Can you work these out from the model? Positions are in its coordinate system, mm. Face numbers are marked on the shaded views. A direction names the side the tool comes from. Give positions to 0.01 mm unless a question says otherwise; leave off trailing zeros. Loops run counter-clockwise (first coordinate to the right, second up) from the corner with the lowest first, then second, coordinate; pieces in that order, holes last. Notation, with made-up numbers: (67, 82) - (119, 82) arc R20 cw to (119, 91) - close; hole circle Ø1 at (65, 10.25). An arc over 180 degrees is marked (long way). Answer as a JSON object with one key per item and string values.
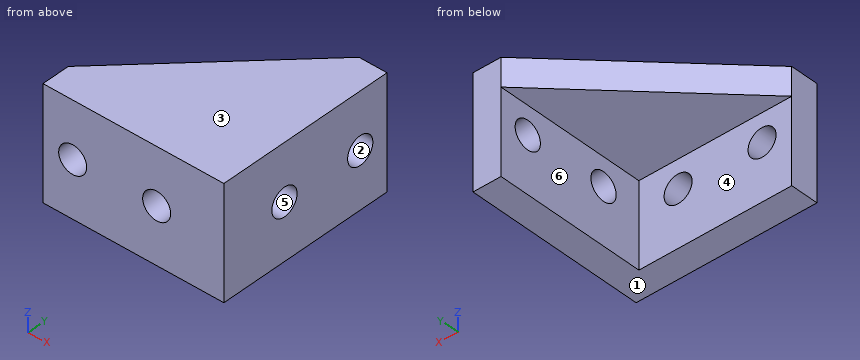
Autodesk Inventor part; units mm, degrees
ref_plane "YZ Plane" through (0, 0, 0) normal (1, 0, 0) x (0, 1, 0)
ref_plane "XZ Plane" through (0, 0, 0) normal (0, 1, 0) x (-1, 0, 0)
ref_plane "XY Plane" through (0, 0, 0) normal (0, 0, 1) x (1, 0, 0)
sketch "Sketch1" plane through (0, 0, 0) normal (0, 0, 1) x (1, 0, 0)
  line L0 (0, 0) -> (50, 0)
  line L1 (50, 0) -> (50, 50)
  line L2 (50, 50) -> (0, 0)
  dimension "d0" = 50
  dimension "d1" = 50
extrude "Extrusion1" add sketch "Sketch1" along normal blind 20
sketch "Sketch2" plane through (0, 0, 20) normal (0, 0, 1) x (1, 0, 0)
  line L0 (50, 50) -> (0, 0)
  line L1 (5, 5) -> (45, 5)
  line L2 (45, 5) -> (45, 45)
  line L3 (50, 0) -> (50, 50)
  line L4 (0, 0) -> (50, 0)
  dimension "d4" = 5
  dimension "d5" = 5
extrude "Extrusion2" cut sketch "Sketch2" against normal through all contours L2 L1 L0
extrude "Extrusion3" add sketch "Sketch2" against normal blind 5 contours L2 L1 L0
sketch "Sketch3" plane through (0, 0, 0) normal (0, 0, -1) x (-1, 0, 0)
  line L0 (-12.7, 0) -> (-50, 37.3)
  line L1 (-50, 0) -> (-50, 50)
  line L2 (-60.6675, 53.6604) -> (-50, 37.3)
  line L3 (-60.6675, 53.6604) -> (-37.4752, 61.571)
  line L4 (-37.4752, 61.571) -> (23.8314, -5.4888)
  line L5 (23.8314, -5.4888) -> (-5.9204, -12.6802)
  line L6 (-5.9204, -12.6802) -> (-12.7, 0)
  point P0 (0, 0)
  dimension "d12" = 12.7
  dimension "d13" = 12.7
extrude "Extrusion5" cut sketch "Sketch3" against normal through all
sketch "Sketch5" plane through (45, 5, 0) normal (-1, 0, 0) x (0, 0, 1)
  line L0 (0, 0) -> (0, 27.3)
  line L1 (20, -5) -> (0, -5)
  point P0 (10, 22)
  point P1 (10, 7)
  dimension "d28" = 10
  dimension "d29" = 10
  dimension "d30" = 15
  dimension "d31" = 12
hole "Hole2" at (45, 27, 10) at (45, 12, 10) direction (1, 0, 0) diameter 5 depth 25.4 tip angle 118
sketch "Sketch6" plane through (45, 5, 15) normal (0, 1, 0) x (1, 0, 0)
  line L0 (-27.3, 15) -> (0, 15)
  line L1 (5, 15) -> (5, -5)
  point P0 (-45, 15)
  point P1 (-7, 5)
  point P2 (-22, 5)
  dimension "d39" = 15
  dimension "d40" = 10
  dimension "d41" = 10
  dimension "d42" = 12
hole "Hole3" at (38, 5, 10) at (23, 5, 10) direction (0, -1, 0) diameter 5 depth 25.4 tip angle 118
sketch "Sketch7" plane through (0, 0, 0) normal (0, 0, -1) x (-1, 0, 0)
  line L0 (-17.7, 5) -> (-17.7, 0)
  line L1 (-12.7, 0) -> (-50, 0)
  line L2 (-17.7, 0) -> (-12.7, 0)
  line L3 (-12.7, 0) -> (-17.7, 5)
  line L4 (-12.7, 0) -> (-17.7, 5)
  line L5 (-45, 32.3) -> (-50, 32.3)
  line L6 (-50, 0) -> (-50, 37.3)
  line L7 (-50, 32.3) -> (-50, 37.3)
  line L8 (-50, 37.3) -> (-45, 32.3)
  line L9 (-45, 32.3) -> (-50, 37.3)
  point P0 (0, 0)
extrude "Extrusion6" cut sketch "Sketch7" against normal blind 25.4
properties part number "corners"
1) Imagine slicing it at C-C on z = 9.5. Write out the boundary of the cut face in (x, y).
Check sheet entries:
{"outline": "(17.7, 0) - (20.55, 0) - (20.55, 5) - (17.7, 5) - close; (25.45, 0) - (35.55, 0) - (35.55, 5) - (25.45, 5) - close; (40.45, 0) - (50, 0) - (50, 9.55) - (45, 9.55) - (45, 5) - (40.45, 5) - close; (45, 14.45) - (50, 14.45) - (50, 24.55) - (45, 24.55) - close; (45, 29.45) - (50, 29.45) - (50, 32.3) - (45, 32.3) - close"}
2) Imagine slicing it at B-B on x = 38. Write out the boundary of the cut face in (y, z).
Check sheet entries:
{"outline": "(0, 0) - (5, 0) - (5, 7.5) - (0, 7.5) - close; (0, 12.5) - (5, 12.5) - (5, 15) - (25.3, 15) - (25.3, 20) - (0, 20) - close"}
3) I'm going to push flat-ended pins straight in: P1, Ø6, axis at y = 16.5, z = 6.5, coming from the -X side; P2, Ø1.5, axis at x = 24.5, y = 12.5, coming from the -Z side; P3, Ø12, axis at y = 18.5, z = 17.5, coming from the -X side. Where does each tip first touch, or does it pass through?
Check sheet entries:
{"P1": "x = 45", "P2": "z = 15", "P3": "x = 25.2"}
4) I need wall thicknesses on L1, parallel to X at y = 3.6, z = 10; L2, parallel to Y at x = 46.95, z = 10; L3, parallel to Z at x = 47.75, y = 12. Which ranges of each line are inside material? Lowest first, please.
Check sheet entries:
{"L1": "17.7 to 20.5, 25.5 to 35.5, 40.5 to 50", "L2": "0 to 9.5, 14.5 to 24.5, 29.5 to 32.3", "L3": "0 to 7.5, 12.5 to 20"}
5) Which directions (+Z, -Z, +X, -X, +Y, -Y) give clear straight access to the entire face, cutting with the end or side of a thin tool? Please do the marked faces 5 and 6.
Check sheet entries:
{"face 5": "+X, -X", "face 6": "-Z, -X, +Y"}
6) If we mould it in two halves opening along Z, with no side actions, what happens to the marked faces 1, 2, 3 and 4? For each: released by +Z, released by -Z, zero draft, split by the parting line, or undercut.
Check sheet entries:
{"face 1": "released by -Z", "face 2": "undercut", "face 3": "released by +Z", "face 4": "zero draft"}
7) Imagine slicing it at A-A on y = 29. Write out the boundary of the cut face in (x, z).
Check sheet entries:
{"outline": "(41.7, 15) - (45, 15) - (45, 11.5) - (50, 11.5) - (50, 20) - (41.7, 20) - close; (45, 0) - (50, 0) - (50, 8.5) - (45, 8.5) - close"}
8) Imagine slicing it at D-D on y = 3.5. Write out the boundary of the cut face in (x, z).
Check sheet entries:
{"outline": "(17.7, 0) - (50, 0) - (50, 20) - (17.7, 20) - close; hole circle Ø5 at (23, 10); hole circle Ø5 at (38, 10)"}
